Autodesk Inventor part; units mm, degrees
ref_plane "YZ Plane" through (0, 0, 0) normal (1, 0, 0) x (0, 1, 0)
ref_plane "XZ Plane" through (0, 0, 0) normal (0, 1, 0) x (-1, 0, 0)
ref_plane "XY Plane" through (0, 0, 0) normal (0, 0, 1) x (1, 0, 0)
sketch "Sketch1" plane through (0, 0, 0) normal (0, 0, 1) x (1, 0, 0)
  line L0 (0, 0) -> (12.7, 0)
  line L1 (12.7, 0) -> (12.7, 67.5875)
  line L2 (12.7, 67.5875) -> (0, 67.5875)
  line L3 (0, 67.5875) -> (0, 0)
  dimension "d0" = 67.5875
  dimension "d1" = 12.7
extrude "Extrusion1" add sketch "Sketch1" along normal blind 168.3364
sketch "Sketch2" plane through (12.7, 0, 0) normal (1, 0, 0) x (0, 0, -1)
  line L0 (0, 0) -> (-168.3364, 0)
  line L1 (-99.8382, 5.715) -> (-99.8382, 5.715)
  line L2 (-168.3364, 67.5875) -> (-168.3364, 0)
  circle A0 centre (-99.8382, 0) radius 3.9688
  circle A1 centre (-68.8382, 0) radius 3.9688
  point P0 (-103.0132, 0)
  dimension "d9" = 7.9375
  dimension "d10" = 31
  dimension "d11" = 68.4982
extrude "Extrusion3" cut sketch "Sketch2" against normal through all
equation "\"d0\" = BaseSupportHeight"
equation "\"d1\" = BaseSupportThickness"
equation "\"d2\" = BaseSideLength"
equation "\"d10\" = HoleSpacing"
properties part number "Robot-Base-Support" material "Wood (Birch)"
The model under review builds one solid part; all positions refer to its coordinate system, in mm. Round coordinates to 2 decimals unless told otherwise and drop trailing zeros. Answer as a JSON object with one key per item and string values. Group by question number.
1) Mouldability with a two-part tool opening along Z and no side actions: class faces 1 (the face through (6, 34, 168.336)), 2 (the face through (6, 0, 32)), 3 (the face through (6.439, 3.968, 99.751)) as released by +Z, released by -Z, zero draft, split by the parting line, or undercut.
2) For line 1 (Z direction, x = 11.5, y = 3), list the stretches that pass through material, from the lowest coordinate up. Write a range as [from, to].
3) For pin 1 Ø4 at (y, z) = (28, 63) entering from -X, flat-tipped, find the tip position at first contact; note if it passes through.
Result set:
{
 "1": {"face 1": "released by +Z", "face 2": "zero draft", "face 3": "undercut"},
 "2": {"line 1": "[0, 66.24], [71.44, 97.24], [102.44, 168.34]"},
 "3": {"pin 1": "x = 0"}
}
